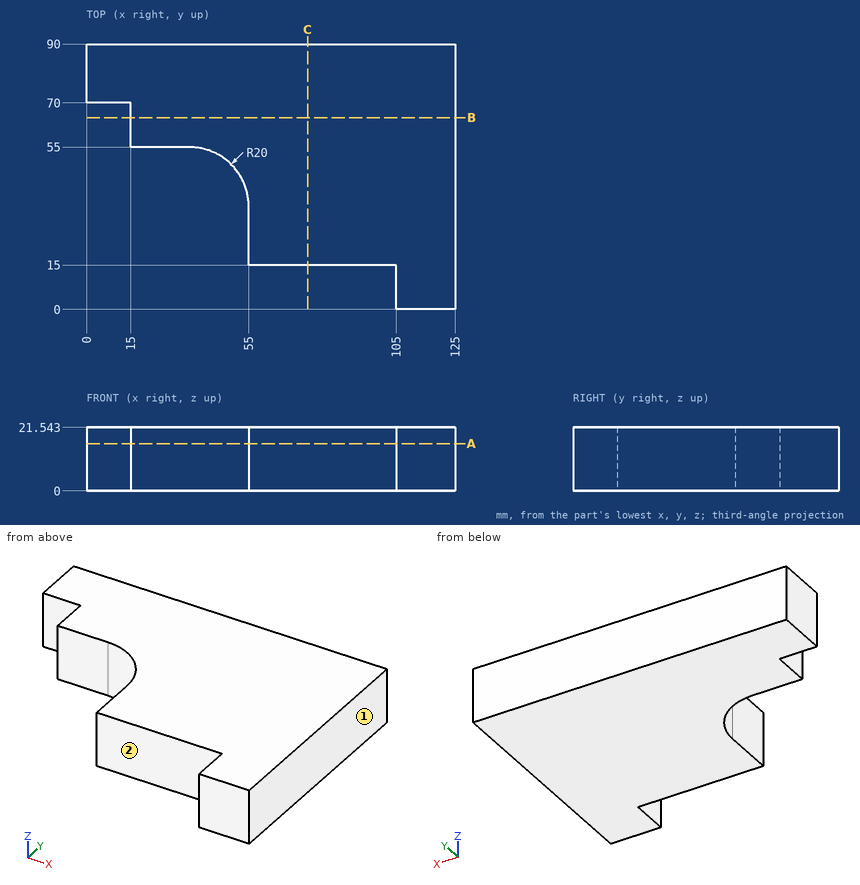
Print and shaded views of the part. All mm, measured from the part's lowest x, y and z. A direction names the side the tool comes from. Round coordinates to 2 decimals unless told otherwise and drop trailing zeros. Order: outer loops, then holes, each group sorted by start corner. A loop starts at its lowest first (then second) coordinate and runs counter-clockwise, first axis right, second up. Notation, with made-up numbers: (-17, 68) - (13, 68) arc R16 cw to (13, 83) - close; hole circle Ø10 at (85, 15). An arc over 180 degrees is marked (long way). Use a Markdown table: item, result.
1) Saw through at C-C on x = 75. Write the cut outline in (y, z).
Recorded:
| item | result |
|---|---|
| outline | (15, 0) - (90, 0) - (90, 21.54) - (15, 21.54) - close |
2) Flat gauge pins, fed straight in: pin 1 Ø7.5 at (x, z) = (7.5, 9.5) entering from -Y; pin 2 Ø1.5 at (x, y) = (88, 13) entering from +Z; pin 3 Ø6.5 at (x, z) = (73.5, 6.5) entering from -Y; pin 4 Ø12 at (y, z) = (35, 6) entering from -X. Where does each tip first touch, or does it go through?
Recorded:
| item | result |
|---|---|
| pin 1 | stops at y = 70 |
| pin 2 | passes through |
| pin 3 | stops at y = 15 |
| pin 4 | stops at x = 54.08 |
3) Saw through at A-A on z = 16. Write the cut outline in (x, y).
Recorded:
| item | result |
|---|---|
| outline | (0, 70) - (15, 70) - (15, 55) - (35, 55) arc R20 cw to (55, 35) - (55, 15) - (105, 15) - (105, 0) - (125, 0) - (125, 90) - (0, 90) - close |
4) Saw through at B-B on y = 65. Write the cut outline in (x, z).
Recorded:
| item | result |
|---|---|
| outline | (15, 0) - (125, 0) - (125, 21.54) - (15, 21.54) - close |
5) Tool access for the marked faces 1 and 2: list every direction of +Z, -Z, +X, -X, +Y, -Y with a clear straight run to the whole face (end or side of a thin tool).
Recorded:
| item | result |
|---|---|
| face 1 | +Z, -Z, +X, +Y, -Y |
| face 2 | +Z, -Z, -X, -Y |
6) Wall check: L1, parallel to Y at x = 69, z = 3.5; L2, parallel to X at y = 69.5, z = 4.75; L3, parallel to Y at x = 14.5, z = 17.5. Give the ranges that are in metal, low to high.
Recorded:
| item | result |
|---|---|
| L1 | y = 15 to 90 |
| L2 | x = 15 to 125 |
| L3 | y = 70 to 90 |
